Input: part model. Units: mm. Frame: model coordinates. A direction names the side the tool comes from. Coordinates: 2 decimals unless noted, no trailing zeros. Loops run counter-clockwise (first coordinate to the right, second up) from the corner with the lowest first, then second, coordinate; pieces in that order, holes last. Notation, with made-up numbers: (70, 59) -> (98, 59) arc R17 cw to (98, 72) -> close; hole circle Ø1 at (29.25, -35). An arc over 180 degrees is marked (long way). Answer as a JSON object with one key per item and string values.
from build123d import *

# Parameters (mm, degrees)
EXTRUDE_1_DEPTH     = 24.5
SKETCH_2_R          = 0.75
CUT_EXTRUDE_1_DEPTH = 5
SKETCH_3_R          = 0.75
CUT_EXTRUDE_2_DEPTH = 5
SKETCH_4_W          = 3
SKETCH_4_H          = 18.5
CUT_EXTRUDE_3_DEPTH = 5
SKETCH_5_W          = 18.5
SKETCH_5_H          = 3
CUT_EXTRUDE_4_DEPTH = 5


with BuildPart() as part:
    # 草圖1 → 填料-伸長1 (new body)
    with BuildSketch(Plane.XY):
        Polygon((0, 0), (0, 21.2), (4.9, 21.2), (4.9, 4.9), (21.2, 4.9), (21.2, 0), align=None)
    extrude(amount=EXTRUDE_1_DEPTH)

    # 草圖2 → 除料-伸長1 (cut)
    with BuildSketch(Plane(origin=(21.2, 0, 0), x_dir=(0, 0, -1), z_dir=(1, 0, 0))):
        with Locations(Location((-6.1, 2.45, 0), (0, 0, 90))):
            Circle(SKETCH_2_R)
        with Locations(Location((-18.4, 2.45, 0), (0, 0, 90))):
            Circle(SKETCH_2_R)
    extrude(amount=-CUT_EXTRUDE_1_DEPTH, mode=Mode.SUBTRACT)

    # 草圖3 → 除料-伸長2 (cut)
    with BuildSketch(Plane(origin=(0, 21.2, 0), x_dir=(1, 0, 0), z_dir=(0, 1, 0))):
        with Locations(Location((2.45, -6.1, 0), (0, 0, 180))):
            Circle(SKETCH_3_R)
        with Locations(Location((2.45, -18.4, 0), (0, 0, 180))):
            Circle(SKETCH_3_R)
    extrude(amount=-CUT_EXTRUDE_2_DEPTH, mode=Mode.SUBTRACT)

    # 草圖4 → 除料-伸長3 (cut)
    with BuildSketch(Plane(origin=(0, 4.9, 0), x_dir=(-1, 0, 0), z_dir=(0, 1, 0))):
        with Locations((-9.4, 12.25)):
            Rectangle(SKETCH_4_W, SKETCH_4_H)
    extrude(amount=-CUT_EXTRUDE_3_DEPTH, mode=Mode.SUBTRACT)

    # 草圖5 → 除料-伸長4 (cut)
    with BuildSketch(Plane(origin=(4.9, 0, 0), x_dir=(0, 0, -1), z_dir=(1, 0, 0))):
        with Locations((-12.25, 9.4)):
            Rectangle(SKETCH_5_W, SKETCH_5_H)
    extrude(amount=-CUT_EXTRUDE_4_DEPTH, mode=Mode.SUBTRACT)


solid = part.part
1. Pin query (flat end, axial travel): P1, Ø0.9, axis at y = 2.45, z = 18.4, coming from the +X side; P2, Ø0.8, axis at x = 2.5, z = 6, coming from the +Y side; P3, Ø2, axis at y = 16, z = 16.5, coming from the +X side. Return the tip coordinate at first contact, or that it passes through.
Reply:
{"P1": "stops at x = 16.2", "P2": "stops at y = 16.2", "P3": "stops at x = 4.9"}
2. Section query B-B (y = 2.45). Return loops of the section in (x, z), plus the area to 3 significant figures.
Reply:
{"outline": "(0, 0) -> (21.2, 0) -> (21.2, 5.35) -> (16.2, 5.35) -> (16.2, 6.85) -> (21.2, 6.85) -> (21.2, 17.65) -> (16.2, 17.65) -> (16.2, 19.15) -> (21.2, 19.15) -> (21.2, 24.5) -> (0, 24.5) -> close; hole (7.9, 3) -> (10.9, 3) -> (10.9, 21.5) -> (7.9, 21.5) -> close", "area": "449 mm2"}
3. Section query C-C (x = 19). Return loops of the section in (y, z).
Reply:
{"outline": "(0, 0) -> (4.9, 0) -> (4.9, 24.5) -> (0, 24.5) -> close; hole circle Ø1.5 at (2.45, 6.1); hole circle Ø1.5 at (2.45, 18.4)"}
4. Line query: line 1 along Z through (x, y) = (2.45, 17.9); line 2 along X through (y, z) = (2.5, 19); line 3 along X through (y, z) = (3.25, 7.5). Output: solid intervals per line, ascending.
Reply:
{"line 1": "z = 0 to 5.35, 6.85 to 17.65, 19.15 to 24.5", "line 2": "x = 0 to 7.9, 10.9 to 16.2", "line 3": "x = 0 to 7.9, 10.9 to 21.2"}
5. Access query for faces 5 (the face through (2, 9, 21.5)), 6 (the face through (9, 2, 3)), 7 (the face through (2.548, 18.735, 19.144)), 8 (the face through (13, 4.9, 12)), 9 (the face through (16.2, 2.4, 18.4)). Directions: +Z, -Z, +X, -X, +Y, -Y. A direction counts if a zero-diameter tool reaches every point of the face in a straight line with its end or side. Return the directions, or none.
Reply:
{"face 5": "+X, -X", "face 6": "+Y, -Y", "face 7": "+Y", "face 8": "+Z, -Z, +X, +Y", "face 9": "+X"}
6. Section query A-A (z = 18.4). Return loops of the section in (x, y).
Reply:
{"outline": "(0, 0) -> (7.9, 0) -> (7.9, 4.9) -> (4.9, 4.9) -> (4.9, 7.9) -> (0, 7.9) -> close; (0, 10.9) -> (4.9, 10.9) -> (4.9, 21.2) -> (3.2, 21.2) -> (3.2, 16.2) -> (1.7, 16.2) -> (1.7, 21.2) -> (0, 21.2) -> close; (10.9, 0) -> (21.2, 0) -> (21.2, 1.7) -> (16.2, 1.7) -> (16.2, 3.2) -> (21.2, 3.2) -> (21.2, 4.9) -> (10.9, 4.9) -> close"}
7. Mould query, pull axis Z, two halves, no side actions, for faces 1 (the face through (2, 16.2, 6)), 2 (the face through (6, 4, 24.5)), 3 (the face through (6, 4, 0)), 4 (the face through (13, 0, 12)). Classes: pulls with the +Z half, pulls with the -Z half, needs draft (parallel to the pull), parting line crosses it, or undercut.
Reply:
{"face 1": "undercut", "face 2": "pulls with the +Z half", "face 3": "pulls with the -Z half", "face 4": "needs draft"}
